Could you check a few things on this model? Use its own coordinates, in mm. Face numbers are marked on the shaded views. A direction names the side the tool comes from. Round coordinates to 2 decimals unless told otherwise and drop trailing zeros. Write each loop counter-clockwise with the first axis right and the second up, starting at its lowest first coordinate (ties: lowest second). Pieces come first, ordered by that corner, then holes. Notation, with made-up numbers: (54, 41.25) -> (82, 41.25) arc R21 ccw to (82, 76.25) -> close; hole circle Ø9 at (56.5, -23.75). An arc over 180 degrees is marked (long way). Answer in a Markdown table with one row per item.
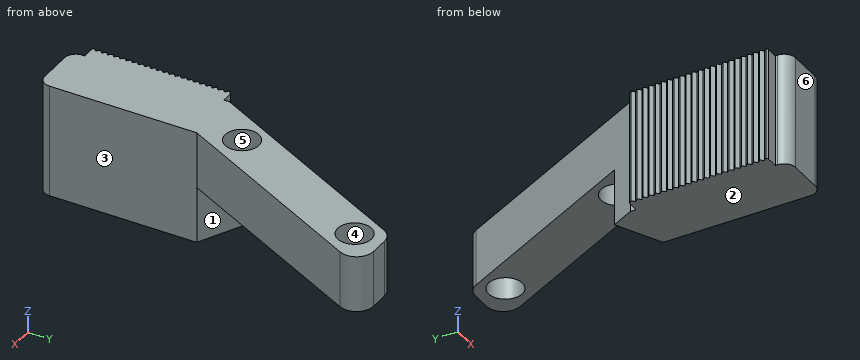
from build123d import *

# Parameters (mm, degrees)
SKETCH2_R           = 1.5
BOSS_EXTRUDE1_DEPTH = 10
SKETCH4_W           = 5
SKETCH4_H           = 22.360679775
CUT_EXTRUDE1_DEPTH  = 10
FILLET1_R           = 1.5
FILLET2_R           = 1
BOSS_EXTRUDE2_DEPTH = 10


with BuildPart() as part:
    # Sketch2 → Boss-Extrude1 (new body)
    with BuildSketch(Plane.XY):
        Polygon((0, 0), (-5, 0), (-15, -20), (-15, -34), (-10, -34), (-10, -20), align=None)
        with Locations((-3.855019194, -2.5)):
            Circle(SKETCH2_R, mode=Mode.SUBTRACT)
        with Locations((-10.857407264, -16.5)):
            Circle(SKETCH2_R, mode=Mode.SUBTRACT)
    extrude(amount=BOSS_EXTRUDE1_DEPTH)

    # Sketch4 → Cut-Extrude1 (cut)
    with BuildSketch(Plane(origin=(0, 0, 0), x_dir=(0, 0, -1), z_dir=(0.894427191, -0.447213595, 0))):
        with Locations((-2.5, -11.180339888)):
            Rectangle(SKETCH4_W, SKETCH4_H)
    extrude(amount=-CUT_EXTRUDE1_DEPTH, mode=Mode.SUBTRACT)

    # Fillet1
    fillet1_edges = [part.edges().sort_by_distance(p)[0] for p in [
        (-5, 0, 7.5),
        (0, 0, 7.5),
    ]]
    fillet(fillet1_edges, radius=FILLET1_R)

    # Fillet2
    fillet2_edges = [part.edges().sort_by_distance(p)[0] for p in [
        (-15, -34, 5),
        (-10, -34, 5),
    ]]
    fillet(fillet2_edges, radius=FILLET2_R)

    # Sketch5 → Boss-Extrude2 (add)
    with BuildSketch(Plane.XY.offset(10)):
        Polygon((-15, -20.5), (-16, -20.5), (-16.270880122, -20.770880122), (-16, -21.041760245), (-16.270880122, -21.312640367), (-16, -21.58352049), (-16.270880122, -21.854400612), (-16, -22.125280734), (-16.270880122, -22.396160857), (-16, -22.667040979), (-16.270880122, -22.937921102), (-16, -23.208801224), (-16.270880122, -23.479681346), (-16, -23.750561469), (-16.270880122, -24.021441591), (-16, -24.292321714), (-16.270880122, -24.563201836), (-16, -24.834081958), (-16.270880122, -25.104962081), (-16, -25.375842203), (-16.270880122, -25.646722326), (-16, -25.917602448), (-16.270880122, -26.188482571), (-16, -26.459362693), (-16.270880122, -26.730242815), (-16, -27.001122938), (-16.270880122, -27.27200306), (-16, -27.542883183), (-16.270880122, -27.813763305), (-16, -28.084643427), (-16.270880122, -28.35552355), (-16, -28.626403672), (-16.270880122, -28.897283795), (-16, -29.168163917), (-16.270880122, -29.439044039), (-16, -29.709924162), (-16.270880122, -29.980804284), (-16, -30.251684407), (-16.270880122, -30.522564529), (-16, -30.793444651), (-16.270880122, -31.064324774), (-16, -31.335204896), (-16.270880122, -31.606085019), (-16, -31.876965141), (-16.270880122, -32.147845263), (-16, -32.418725386), (-16.270880122, -32.689605508), (-16.070783647, -32.79), (-15, -32.79), align=None)
    extrude(amount=-BOSS_EXTRUDE2_DEPTH)


solid = part.part
1) Imagine slicing it at B-B, the plane x = -4.5. Please give me the cut outline in (y, z).
Findings:
| item | result |
|---|---|
| outline | (-9, 5) -> (-3.85, 5) -> (-3.85, 10) -> (-9, 10) -> close; (-1.15, 5) -> (-0.06, 5) -> (-0.06, 10) -> (-1.15, 10) -> close |
2) Please list where these lines run through material, in increasing order: line 1 (X direction, y = -16.5, z = 8.2); line 2 (X direction, y = -17.5, z = 9.25); line 3 (Y direction, x = -10.25, z = 8.75).
Findings:
| item | result |
|---|---|
| line 1 | x = -13.25 to -12.36, -9.36 to -8.25 |
| line 2 | x = -13.75 to -11.98, -9.74 to -8.75 |
| line 3 | y = -33.66 to -17.87, -15.13 to -10.5 |
3) For the marked faces 1 and 2, which set-ups out of +Z, -Z, +X, -X, +Y, -Y let a thin tool reach every point of the face, with its end or its side?
Findings:
| item | result |
|---|---|
| face 1 | -Z, +X, +Y |
| face 2 | -Z, +X, -X, +Y, -Y |
4) Thinking about a two-plate mould opening in X: for the marked faces 3, 4, 5 and 6, which applies, +X half, -X half, draft (parallel to the pull), parting line (faces both ways), or undercut?
Findings:
| item | result |
|---|---|
| face 3 | +X half |
| face 4 | undercut |
| face 5 | undercut |
| face 6 | draft |
5) Imagine slicing it at C-C, the plane z = 5.5. Count the separate pieces of the cut face and the enclosed holes in it, plus the area to 3 significant figures.
Findings:
| item | result |
|---|---|
| separate pieces | 1 |
| enclosed holes | 2 |
| area | 168 mm^2 |
6) For pin 1 (5 mm diameter, centred on y = -25.5, z = 4.5, fed in from +X); pin 2 (2 mm diameter, centred on y = -6.5, z = 5.5, fed in from +X); pin 3 (6 mm diameter, centred on x = -7.5, z = 8.5, fed in from +Y), each with a flat end and sliding along its axis, tell me the tip position at first contact or that it passes through.
Findings:
| item | result |
|---|---|
| pin 1 | stops at x = -10 |
| pin 2 | stops at x = -2.75 |
| pin 3 | stops at y = -0.06 |
7) Imagine slicing it at D-D, the plane y = -6. Please give me the cut outline in (x, z).
Findings:
| item | result |
|---|---|
| outline | (-8, 5) -> (-3, 5) -> (-3, 10) -> (-8, 10) -> close |
8) Imagine slicing it at A-A, the plane y = -2.5. Please give me the cut outline in (x, z).
Findings:
| item | result |
|---|---|
| outline | (-6.25, 5) -> (-5.36, 5) -> (-5.36, 10) -> (-6.25, 10) -> close; (-2.36, 5) -> (-1.25, 5) -> (-1.25, 10) -> (-2.36, 10) -> close |
